```python
from build123d import *

# Parameters (mm, degrees)
CROQUIS2_R              = 3
SALIENTE_EXTRUIR1_DEPTH = 17.61
CROQUIS3_R              = 7
CROQUIS3_R_2            = 3
SALIENTE_EXTRUIR2_DEPTH = 1
CHAFL_N1_SIZE           = 0.25
CROQUIS4_R              = 14
SALIENTE_EXTRUIR3_DEPTH = 1.5
CHAFL_N2_SIZE           = 0.7
REDONDEO3_R             = 4.4
CROQUIS6_R              = 1.25
CROQUIS6_R_2            = 0.75
CORTAR_EXTRUIR1_DEPTH   = 0.2
REDONDEO4_R             = 0.2
REDONDEO5_R             = 0.2
SALIENTE_EXTRUIR4_START = 2.36
CROQUIS7_R              = 5.175
CROQUIS7_R_2            = 3
SALIENTE_EXTRUIR4_DEPTH = 2.36


with BuildPart() as part:
    # Croquis1 → Revolución1 (revolve)
    with BuildSketch(Plane.XY, mode=Mode.PRIVATE) as revoluci_n1_sk:
        Polygon((-3, 0.98), (-7.5, 0.98), (-14, 0), (0, 0), (0, 82.891267921), (-3, 82.891267921), align=None)
    revolve(revoluci_n1_sk.sketch.rotate(Axis((0, 0, 0), (0, 1, 0)), 270), axis=Axis((0, 0, 0), (0, 1, 0)))

    # Croquis2 → Saliente-Extruir1 (add)
    with BuildSketch(Plane(origin=(0, 82.891267921, 0), x_dir=(1, 0, 0), z_dir=(0, 1, 0))):
        with Locations(Location((0, 0, 0), (0, 0, 90))):
            Circle(CROQUIS2_R)
    extrude(amount=SALIENTE_EXTRUIR1_DEPTH)

    # Croquis3 → Saliente-Extruir2 (add)
    with BuildSketch(Plane(origin=(0, 99.501267921, 0), x_dir=(1, 0, 0), z_dir=(0, 1, 0))):
        with Locations(Location((0, 0, 0), (0, 0, 90))):
            Circle(CROQUIS3_R)
        with Locations(Location((0, 0, 0), (0, 0, 90))):
            Circle(CROQUIS3_R_2, mode=Mode.SUBTRACT)
    extrude(amount=SALIENTE_EXTRUIR2_DEPTH)

    # Chaflán1
    chafl_n1_edges = [part.edges().sort_by_distance(p)[0] for p in [
        (0, 99.501267921, 7),
        (0, 100.501267921, 7),
    ]]
    chamfer(chafl_n1_edges, length=CHAFL_N1_SIZE)

    # Croquis4 → Saliente-Extruir3 (add)
    with BuildSketch(Plane.XZ):
        with Locations(Location((0, 0, 0), (0, 0, 270))):
            Circle(CROQUIS4_R)
    extrude(amount=SALIENTE_EXTRUIR3_DEPTH)

    # Chaflán2
    chafl_n2_edges = [part.edges().sort_by_distance(p)[0] for p in [
        (0, -1.5, 14),
    ]]
    chamfer(chafl_n2_edges, length=CHAFL_N2_SIZE)

    # Redondeo3
    redondeo3_edges = [part.edges().sort_by_distance(p)[0] for p in [
        (0, 0.98, 3),
    ]]
    fillet(redondeo3_edges, radius=REDONDEO3_R)

    # Croquis5 → Cortar-Revolución1 (revolve, cut)
    with BuildSketch(Plane(origin=(0, 0, 0), x_dir=(0, 0, -1), z_dir=(1, 0, 0)), mode=Mode.PRIVATE) as cortar_revoluci_n1_sk:
        Polygon((-7.5, 0.98), (-14, 0), (-14, -0.4), (-7.5, 0.58264143), align=None)
    revolve(cortar_revoluci_n1_sk.sketch.rotate(Axis((0, 0, 0), (0, 1, 0)), 180), axis=Axis((0, 0, 0), (0, 1, 0)), mode=Mode.SUBTRACT)

    # Croquis6 → Cortar-Extruir1 (cut)
    with BuildSketch(Plane(origin=(0, 100.501267921, 0), x_dir=(1, 0, 0), z_dir=(0, 1, 0))):
        with Locations(Location((0, 0, 0), (0, 0, 270))):
            Circle(CROQUIS6_R)
        with Locations(Location((0, 0, 0), (0, 0, 270))):
            Circle(CROQUIS6_R_2, mode=Mode.SUBTRACT)
    extrude(amount=-CORTAR_EXTRUIR1_DEPTH, mode=Mode.SUBTRACT)

    # Redondeo4
    redondeo4_edges = [part.edges().sort_by_distance(p)[0] for p in [
        (0, 100.301267921, -1.25),
    ]]
    fillet(redondeo4_edges, radius=REDONDEO4_R - 0.0001)  # a hair under: the kernel refuses the full size

    # Redondeo5
    redondeo5_edges = [part.edges().sort_by_distance(p)[0] for p in [
        (0, 100.501267921, -0.75),
    ]]
    fillet(redondeo5_edges, radius=REDONDEO5_R - 0.0001)  # a hair under: the kernel refuses the full size

    # Croquis7 → Saliente-Extruir4 (add)
    with BuildSketch(Plane.XZ.offset(-99.501267921).offset(SALIENTE_EXTRUIR4_START)):
        with Locations(Location((0, 0, 0), (0, 0, 90))):
            Circle(CROQUIS7_R)
        with Locations(Location((0, 0, 0), (0, 0, 270))):
            Circle(CROQUIS7_R_2, mode=Mode.SUBTRACT)
    extrude(amount=-SALIENTE_EXTRUIR4_DEPTH)


solid = part.part
```
Work out the finished part from the listing and answer in its coordinate system (mm). A direction names the side the tool comes from. Give positions to 0.01 mm unless a question says otherwise; leave off trailing zeros. Order: outer loops, then holes, each group sorted by start corner. A loop starts at its lowest first (then second) coordinate and runs counter-clockwise, first axis right, second up. Notation, with made-up numbers: M 22.5,-19 L 54.5,-19 A19 cw 54.5,-1 Z; hole C -20,37 d5. An arc over 180 degrees is marked long. Return JSON: item names as keys, results as strings.
1) A tool of negligible diameter and unlimited length cuts with its end or side. For faces 5 (the flat face through (5, 99.501, 2)), 6 (the cylindrical face through (-6.324, 0.784, -4.032)), 7 (the cylindrical face through (-13.67, -0.6, 3.03)), from which of +Z, -Z, +X, -X, +Y, -Y can it reach the whole face along a straight path? Write none if from no direction.
Resolved:
{"face 5": "none", "face 6": "+Y", "face 7": "+Y, -Y"}
2) Straight lines are drawn through the part: line 1 along Y through (x, z) = (5.75, 1); line 2 along X through (y, z) = (25, 0.25); line 3 along Z through (x, y) = (0, 17.5). For each, find the intervals that lie inside material, in ascending order. Write a range as [from, to].
Resolved:
{"line 1": "[-1.5, 1.27], [99.5, 100.5]", "line 2": "[-2.99, 2.99]", "line 3": "[-3, 3]"}
3) Each of these flat-tipped pins is pushed along its axis until it touches: pin 1 (6 mm diameter, centred on y = 54, z = -7, fed in from +X); pin 2 (8 mm diameter, centred on y = 89, z = 0, fed in from -X); pin 3 (2 mm diameter, centred on x = -3.5, y = 47, fed in from -Z). Where does it stop, or does it pass through?
Resolved:
{"pin 1": "through", "pin 2": "x = -3", "pin 3": "z = -1.66"}
4) For a pull along Y with two mould halves and no side action, classify faces 1 (the cylindrical face through (-0.9, 50.62, -2.86)), 2 (the cylindrical face through (3.149, 98.305, -4.107)), 3 (the cylindrical face through (6.834, 99.998, 1.517)), 4 (the conical face through (7.63, 0.535, 1.694)) as +Y half, -Y half, draft (parallel to the pull), parting line (faces both ways), or undercut.
Resolved:
{"face 1": "undercut", "face 2": "undercut", "face 3": "draft", "face 4": "+Y half"}
5) Section A-A, the plane y = 72 is taken. Write down the section's boundary in (x, z).
Resolved:
{"outline": "C 0,0 d6"}
